Design review of the part built by this model. Coordinates are the model's own, in mm. A direction names the side the tool comes from. Give positions to 0.01 mm unless a question says otherwise; leave off trailing zeros. Write each loop counter-clockwise with the first axis right and the second up, starting at its lowest first coordinate (ties: lowest second). Pieces come first, ordered by that corner, then holes. Notation, with made-up numbers: (-4.5, 6) -> (29.5, 6) arc R11 ccw to (29.5, 17) -> close; hole circle Ø9 at (71.25, 75). An arc over 180 degrees is marked (long way). Use CSV: the item, a comma, the result in double quotes.
```python
from build123d import *

# Parameters (mm, degrees)
F0_W     = 19.05
F0_H     = 17.78
F1_DEPTH = 50.8
F2_R     = 3.175
F2_R_2   = 6.0964456607
F3_DEPTH = 19.051
F4_R     = 4
F5_DEPTH = 19.05
F6_R     = 5.07999
F7_SIZE  = 1.5


# Not quite as in the source:
# - a fillet or chamfer is up to 0.001 mm smaller than in the source, because OpenCascade refuses the exact size


with BuildPart() as f1:
    # F0 (on Front) → F1 (new body, symmetric)
    with BuildSketch(Plane.XZ):
        Rectangle(F0_W, F0_H)
    extrude(amount=F1_DEPTH, both=True)

    # F2 (on face) → F3 (cut, through all)
    with BuildSketch(Plane.YZ.offset(9.525)):
        with Locations((-45.43298, 0)):
            Circle(F2_R)
        with Locations((45.43298, 0)):
            Circle(F2_R)
        Circle(F2_R_2)
    extrude(amount=-F3_DEPTH, mode=Mode.SUBTRACT)

    # F4 (on face) → F5 (join, through all)
    with BuildSketch(Plane.YZ.offset(9.525)):
        with BuildLine():
            Line((-10.5791, 19.4691), (-10.5791, 8.89))
            Line((-10.5791, 8.89), (10.5791, 8.89))
            Line((10.5791, 8.89), (10.5791, 19.4691))
            ThreePointArc((10.5791, 19.4691), (0, 30.0482), (-10.5791, 19.4691))
        make_face()
        with Locations((0, 19.4691)):
            Circle(F4_R, mode=Mode.SUBTRACT)
        with BuildLine():
            Line((-10.5791, -8.89), (-10.5791, -13.97))
            ThreePointArc((-10.5791, -13.97), (0, -24.5491), (10.5791, -13.97))
            Line((10.5791, -13.97), (10.5791, -8.89))
            Line((10.5791, -8.89), (-10.5791, -8.89))
        make_face()
        with Locations((0, -13.97)):
            Circle(F4_R, mode=Mode.SUBTRACT)
    extrude(amount=-F5_DEPTH)

    # F6 (radius 5.08 in the source; OpenCascade refuses exactly that, so slightly less here)
    f6_edges = [f1.edges().sort_by_distance(p)[0] for p in [
        (0, -10.5791, 8.89),
        (0, 10.5791, 8.89),
        (0, -10.5791, -8.89),
        (0, 10.5791, -8.89),
    ]]
    fillet(f6_edges, radius=F6_R)

    # F7
    f7_edges = [f1.edges().sort_by_distance(p)[0] for p in [
        (9.525, -33.229545, 8.89),
        (9.525, -33.229545, -8.89),
        (-9.525, -33.229545, 8.89),
        (-9.525, -33.229545, -8.89),
        (-9.525, -50.8, 0),
        (-9.525, 50.8, 0),
        (9.525, -50.8, 0),
        (9.525, 50.8, 0),
    ]]
    chamfer(f7_edges, length=F7_SIZE)


solid = f1.part
```
(1) For line 1 along Z through (x, y) = (-4, 0); line 2 along Y through (x, z) = (-8, -17.5); line 3 along Z through (x, y) = (7.75, 36), list the stretches that pass through material, from the lowest coordinate up. Write a range as [from, to].
Established:
line 1,"z = [-24.55, -17.97], [-9.97, -6.1], [6.1, 15.47], [23.47, 30.05]"
line 2,"y = [-9.97, -1.88], [1.88, 9.97]"
line 3,"z = [-8.89, 8.89]"
(2) Mouldability with a two-part tool opening along Y and no side actions: class faces 1 (the face through (0, -50.8, 0)), 2 (the face through (-9.26, 0.21, -23.31)), 3 (the face through (0.133, 5.815, 1.831)), 4 (the face through (0.1, -0.5, -10)) as +Y half, -Y half, draft (parallel to the pull), parting line (faces both ways), or undercut.
Established:
face 1,"-Y half"
face 2,"parting line"
face 3,"undercut"
face 4,"undercut"
(3) Tool access review of faces 5 (the face through (0, 33, 8.89)), 6 (the face through (0, -33, -8.89)), 7 (the face through (-8.43, -11.82, 10.05)), 8 (the face through (0, 33, -8.89)): name each direction out of +Z, -Z, +X, -X, +Y, -Y from which nothing blocks a thin tool from reaching the whole face with its end or side.
Established:
face 5,"+Z, +X, -X, +Y"
face 6,"-Z, +X, -X, -Y"
face 7,"+Z, -X, -Y"
face 8,"-Z, +X, -X, +Y"
(4) Take a section at C-C (z = 0). Write out the cut boundary in (x, y) (3 decimals).
Established:
outline,"(-9.525, -49.3) -> (-8.025, -50.8) -> (8.025, -50.8) -> (9.525, -49.3) -> (9.525, -48.608) -> (-9.525, -48.608) -> close; (-9.525, -42.258) -> (9.525, -42.258) -> (9.525, -6.096) -> (-9.525, -6.096) -> close; (-9.525, 6.096) -> (9.525, 6.096) -> (9.525, 42.258) -> (-9.525, 42.258) -> close; (-9.525, 48.608) -> (9.525, 48.608) -> (9.525, 49.3) -> (8.025, 50.8) -> (-8.025, 50.8) -> (-9.525, 49.3) -> close"
(5) Take a section at D-D (y = 24.5). Write out the cut boundary in (x, z) (3 decimals).
Established:
outline,"(-9.525, -7.39) -> (-8.025, -8.89) -> (8.025, -8.89) -> (9.525, -7.39) -> (9.525, 7.39) -> (8.025, 8.89) -> (-8.025, 8.89) -> (-9.525, 7.39) -> close"
(6) Take a section at B-B (x = -3). State how many separate pieces and enclosed holes the cut face has, then the cut area to 3 significant figures.
Established:
separate pieces,"1"
enclosed holes,"5"
area,"2,230 mm2"
(7) Clearance check with flat-ended pins moving along their axes: pin 1 (5.5 mm diameter, centred on y = 45.43, z = 0, fed in from +X); pin 2 (2.5 mm diameter, centred on x = -1, z = 18, fed in from +Y); pin 3 (8 mm diameter, centred on x = 3.5, y = 36, fed in from +Z); pin 4 (8 mm diameter, centred on x = -1.5, y = 35.5, fed in from -Z). State where each tip first meets the part, or that it passes through.
Established:
pin 1,"passes through"
pin 2,"stops at y = 10.58"
pin 3,"stops at z = 8.89"
pin 4,"stops at z = -8.89"
(8) Take a section at A-A (y = 0). Write out the cut boundary in (x, z) (3 decimals), then the cut area to 3 significant figures.
Established:
outline,"(-9.525, -23.049) -> (-8.025, -24.549) -> (8.025, -24.549) -> (9.525, -23.049) -> (9.525, -17.97) -> (-9.525, -17.97) -> close; (-9.525, -9.97) -> (9.525, -9.97) -> (9.525, -6.096) -> (-9.525, -6.096) -> close; (-9.525, 6.096) -> (9.525, 6.096) -> (9.525, 15.469) -> (-9.525, 15.469) -> close; (-9.525, 23.469) -> (9.525, 23.469) -> (9.525, 28.548) -> (8.025, 30.048) -> (-8.025, 30.048) -> (-9.525, 28.548) -> close"
area,"499 mm2"
